The model under review builds one solid part; all positions refer to its coordinate system, in mm. A direction names the side the tool comes from. Coordinates: 2 decimals unless noted, no trailing zeros. Loops run counter-clockwise (first coordinate to the right, second up) from the corner with the lowest first, then second, coordinate; pieces in that order, holes last. Notation, with made-up numbers: M 16,84.5 L 68,84.5 A25 ccw 68,110.5 Z; hole C 68,0 d10. An arc over 180 degrees is marked long. Write item = value, one per line. Start each with the question number.
Q1. We need section A-A on y = 12. Give the boundary of the cut face in (x, z), and give its area (3 significant figures).
Q2. Clearance check with flat-ended pins moving along their axes: pin 1 Ø5.5 at (y, z) = (26, 26.5) entering from +X; pin 2 Ø4 at (y, z) = (21, -32) entering from -X; pin 3 Ø10.5 at (x, z) = (-17.5, 10) entering from +Y; pin 4 Ø2 at (x, y) = (-64, -3) entering from -Z. State where each tip first meets the part, or that it passes through.
Q3. Mouldability with a two-part tool opening along Z and no side actions: class faces 1 (the face through (24.5, 29.9, 9.8)), 2 (the face through (-65, -2, -27.5)), 3 (the face through (-26.577, 31.774, 32.535)) as released by +Z, released by -Z, zero draft, split by the parting line, or undercut.
Q4. Wall thickness on probe 1 along Y at (x, z) = (27.5, 32.55); probe 2 along X at (y, z) = (30, 33.95); probe 3 along X at (y, z) = (25, 22.5): over which ranges is each line inside the solid? List them lowest first.
Q5. We need section C-C on x = 9. Give the boundary of the cut face in (y, z), and give its area (3 significant figures).
Q6. We need section B-B on x = -69.5. Give the boundary of the cut face in (y, z), and give its area (3 significant figures).
Q7. We need section D-D on z = -7.5. Give the boundary of the cut face in (x, y), and give its area (3 significant figures).
Q8. For faces 4 (the face through (-27, 18, -30)), 5 (the face through (-24.5, 5.1, 9.8)), 6 (the face through (21.466, -2.535, 10.521)), 7 (the face through (-9, 5, 0)), list the 3-axis set-ups (+Z, -Z, +X, -X, +Y, -Y) from which the entire face can be reached by the end or side of a thin tool; tool diameter is ignored.
from build123d import *

# Parameters (mm, degrees)
SKETCH_1_W          = 45
SKETCH_1_H          = 70
SKETCH_1_R          = 21.5
EXTRUDE_1_DEPTH     = 35
SKETCH_2_R          = 21.5
EXTRUDE_2_DEPTH     = 5
SKETCH_3_R          = 2
SKETCH_3_R_2        = 13
CUT_EXTRUDE_1_DEPTH = 10
SKETCH_5_W          = 10
SKETCH_5_H          = 35
EXTRUDE_3_DEPTH     = 5
SKETCH_6_R          = 2
CUT_EXTRUDE_2_DEPTH = 5
EXTRUDE_START       = 5
SKETCH_8_R          = 22.5
SKETCH_8_R_2        = 13
SKETCH_8_R_3        = 2
EXTRUDE_5_DEPTH     = 5
SKETCH_9_R          = 4
CUT_EXTRUDE_3_DEPTH = 5
EXTRUDE_6_DEPTH     = 7
SKETCH_11_W         = 25
SKETCH_11_H         = 15
EXTRUDE_7_DEPTH     = 7
FILLET_1_R          = 4
SKETCH_12_R         = 2.5
CUT_EXTRUDE_4_DEPTH = 10
SKETCH_13_W         = 5
SKETCH_13_H         = 30
EXTRUDE_8_DEPTH     = 35
SKETCH_14_W         = 65
SKETCH_14_H         = 35
EXTRUDE_9_DEPTH     = 5
CUT_EXTRUDE_START   = -5
SKETCH_16_R         = 2
CUT_EXTRUDE_5_DEPTH = 5
SKETCH_18_R         = 3
CUT_EXTRUDE_6_DEPTH = 31


with BuildPart() as part:
    # 草图1 → 凸台-拉伸1 (new body)
    with BuildSketch(Plane(origin=(0, 0, 0), x_dir=(1, 0, 0), z_dir=(0, 1, 0))):
        Rectangle(SKETCH_1_W, SKETCH_1_H)
        with Locations(Location((0, -10, 0), (0, 0, 270))):
            Circle(SKETCH_1_R, mode=Mode.SUBTRACT)
    extrude(amount=EXTRUDE_1_DEPTH)

    # 草图2 → 凸台-拉伸2 (add)
    with BuildSketch(Plane.XZ):
        with Locations(Location((0, 10, 0), (0, 0, 270))):
            Circle(SKETCH_2_R)
    extrude(amount=-EXTRUDE_2_DEPTH)

    # 草图3 → 切除-拉伸1 (cut)
    with BuildSketch(Plane.XZ):
        with Locations(Location((0, -7.5, 0), (0, 0, 270))):
            Circle(SKETCH_3_R)
        with Locations(Location((-17.5, 10, 0), (0, 0, 270))):
            Circle(SKETCH_3_R)
        with Locations(Location((0, 27.5, 0), (0, 0, 270))):
            Circle(SKETCH_3_R)
        with Locations(Location((17.5, 10, 0), (0, 0, 270))):
            Circle(SKETCH_3_R)
        with Locations(Location((0, 10, 0), (0, 0, 270))):
            Circle(SKETCH_3_R_2)
    extrude(amount=-CUT_EXTRUDE_1_DEPTH, mode=Mode.SUBTRACT)

    # 草图5 → 凸台-拉伸3 (add)
    with BuildSketch(Plane(origin=(0, 0, -35), x_dir=(-1, 0, 0), z_dir=(0, 0, -1))):
        with Locations((27.5, 17.5)):
            Rectangle(SKETCH_5_W, SKETCH_5_H)
        with Locations((-27.5, 17.5)):
            Rectangle(SKETCH_5_W, SKETCH_5_H)
    extrude(amount=-EXTRUDE_3_DEPTH)

    # 草图6 → 切除-拉伸2 (cut)
    with BuildSketch(Plane.XY.offset(-30)):
        with Locations((27.5, 30)):
            Circle(SKETCH_6_R)
        with Locations((27.5, 5)):
            Circle(SKETCH_6_R)
        with Locations((-27.5, 30)):
            Circle(SKETCH_6_R)
        with Locations((-27.5, 5)):
            Circle(SKETCH_6_R)
    extrude(amount=-CUT_EXTRUDE_2_DEPTH, mode=Mode.SUBTRACT)

    # 草图8 → 凸台-拉伸5 (add)
    with BuildSketch(Plane.XZ.offset(EXTRUDE_START)):
        with Locations(Location((0, 10, 0), (0, 0, 180))):
            Circle(SKETCH_8_R)
        with Locations(Location((0, 10, 0), (0, 0, 270))):
            Circle(SKETCH_8_R_2, mode=Mode.SUBTRACT)
        with Locations(Location((-17.5, 10, 0), (0, 0, 270))):
            Circle(SKETCH_8_R_3, mode=Mode.SUBTRACT)
        with Locations(Location((0, -7.5, 0), (0, 0, 270))):
            Circle(SKETCH_8_R_3, mode=Mode.SUBTRACT)
        with Locations(Location((17.5, 10, 0), (0, 0, 270))):
            Circle(SKETCH_8_R_3, mode=Mode.SUBTRACT)
        with Locations(Location((0, 27.5, 0), (0, 0, 270))):
            Circle(SKETCH_8_R_3, mode=Mode.SUBTRACT)
    extrude(amount=-EXTRUDE_5_DEPTH)

    # 草图9 → 切除-拉伸3 (cut)
    with BuildSketch(Plane.XZ.offset(5)):
        with Locations(Location((0, 27.5, 0), (0, 0, 270))):
            Circle(SKETCH_9_R)
        with Locations(Location((-17.5, 10, 0), (0, 0, 270))):
            Circle(SKETCH_9_R)
        with Locations(Location((17.5, 10, 0), (0, 0, 270))):
            Circle(SKETCH_9_R)
        with Locations(Location((0, -7.5, 0), (0, 0, 270))):
            Circle(SKETCH_9_R)
    extrude(amount=-CUT_EXTRUDE_3_DEPTH, mode=Mode.SUBTRACT)

    # 草图10 → 凸台-拉伸6 (add)
    with BuildSketch(Plane.XZ.offset(5)):
        with BuildLine():
            Line((-19.899748742, 20.5), (-77, 20.5))
            Line((-77, 20.5), (-77, -12.5))
            Line((-77, -12.5), (0, -12.5))
            ThreePointArc((0, -12.5), (-19.267848868, -1.618950039), (-19.899748742, 20.5))
        make_face()
    extrude(amount=-EXTRUDE_6_DEPTH)

    # 草图11 → 凸台-拉伸7 (add)
    with BuildSketch(Plane.XZ.offset(5)):
        with Locations((-64.5, -20)):
            Rectangle(SKETCH_11_W, SKETCH_11_H)
    extrude(amount=-EXTRUDE_7_DEPTH)

    # 圆角1
    fillet_1_edges = [part.edges().sort_by_distance(p)[0] for p in [
        (-77, -1.5, 20.5),
        (-77, -1.5, -27.5),
        (-52, -1.5, -12.5),
        (-52, -1.5, -27.5),
    ]]
    fillet(fillet_1_edges, radius=FILLET_1_R)

    # 草图12 → 切除-拉伸4 (cut)
    with BuildSketch(Plane.XZ.offset(5)):
        with Locations(Location((-69.5, -15, 0), (0, 0, 270))):
            Circle(SKETCH_12_R)
        with Locations(Location((-69.5, 15, 0), (0, 0, 270))):
            Circle(SKETCH_12_R)
    extrude(amount=-CUT_EXTRUDE_4_DEPTH, mode=Mode.SUBTRACT)

    # 草图13 → 凸台-拉伸8 (add)
    with BuildSketch(Plane(origin=(0, 0, 0), x_dir=(1, 0, 0), z_dir=(0, 1, 0))):
        with Locations((25, -10)):
            Rectangle(SKETCH_13_W, SKETCH_13_H)
        with Locations((-25, -10)):
            Rectangle(SKETCH_13_W, SKETCH_13_H)
    extrude(amount=EXTRUDE_8_DEPTH)

    # 草图14 → 凸台-拉伸9 (add)
    with BuildSketch(Plane.XY.offset(35)):
        with Locations((0, 17.5)):
            Rectangle(SKETCH_14_W, SKETCH_14_H)
    extrude(amount=-EXTRUDE_9_DEPTH)

    # 草图16 → 切除-拉伸5 (cut)
    with BuildSketch(Plane(origin=(0, 0, 30), x_dir=(-1, 0, 0), z_dir=(0, 0, -1)).offset(CUT_EXTRUDE_START)):
        with Locations(Location((-27.5, 30, 0), (0, 0, 180))):
            Circle(SKETCH_16_R)
        with Locations(Location((-27.5, 5, 0), (0, 0, 180))):
            Circle(SKETCH_16_R)
        with Locations(Location((27.5, 30, 0), (0, 0, 180))):
            Circle(SKETCH_16_R)
        with Locations(Location((27.5, 5, 0), (0, 0, 180))):
            Circle(SKETCH_16_R)
    extrude(amount=CUT_EXTRUDE_5_DEPTH, mode=Mode.SUBTRACT)

    # 草图18 → 切除-拉伸6 (cut)
    with BuildSketch(Plane(origin=(0, 0, -5), x_dir=(-1, 0, 0), z_dir=(0, 0, -1))):
        with Locations((27.5, 30)):
            Circle(SKETCH_18_R)
        with Locations((27.5, 5)):
            Circle(SKETCH_18_R)
        with Locations((-27.5, 5)):
            Circle(SKETCH_18_R)
        with Locations((-27.5, 30)):
            Circle(SKETCH_18_R)
    extrude(amount=-CUT_EXTRUDE_6_DEPTH, mode=Mode.SUBTRACT)


solid = part.part
Returned:
q1.outline = M -32.5,-35 L 32.5,-35 L 32.5,-30 L 22.5,-30 L 22.5,-5 L 27.5,-5 L 27.5,25 L 22.5,25 L 22.5,30 L 32.5,30 L 32.5,35 L -32.5,35 L -32.5,30 L -22.5,30 L -22.5,25 L -27.5,25 L -27.5,-5 L -22.5,-5 L -22.5,-30 L -32.5,-30 Z; hole M -7.89,30 A21.5 ccw long 7.89,30 Z
q1.area = 2,210 mm^2
q2.pin_1 = 27.5
q2.pin_2 = -32.5
q2.pin_3 = 35
q2.pin_4 = -27.5
q3.face_1 = undercut
q3.face_2 = released by -Z
q3.face_3 = zero draft
q4.probe_1 = 0 to 3, 7 to 28, 32 to 35
q4.probe_2 = -32.5 to -29.5, -25.5 to 25.5, 29.5 to 32.5
q4.probe_3 = -27.5 to -17.49, 17.49 to 27.5
q5.outline = M -5,-10.62 L 0,-10.62 L 0,-35 L 35,-35 L 35,-9.53 L 5,-9.53 L 5,0.62 L -5,0.62 Z; M -5,19.38 L 5,19.38 L 5,29.53 L 35,29.53 L 35,35 L 0,35 L 0,30.62 L -5,30.62 Z
q5.area = 1,300 mm^2
q6.outline = M -5,-27.5 L 2,-27.5 L 2,-17.5 L -5,-17.5 Z; M -5,-12.5 L 2,-12.5 L 2,12.5 L -5,12.5 Z; M -5,17.5 L 2,17.5 L 2,20.5 L -5,20.5 Z
q6.area = 266 mm^2
q7.outline = M -77,-5 L -4,-5 L -4,0 L -2,0 L -2,5 L -12.49,5 L -12.49,35 L -22.5,35 L -22.5,2 L -77,2 Z; M 2,0 L 4,0 L 4,-5 L 14.14,-5 L 14.14,0 L 22.5,0 L 22.5,35 L 12.49,35 L 12.49,5 L 2,5 Z
q7.area = 1,330 mm^2
q8.face_4 = -X, +Y, -Y
q8.face_5 = -X
q8.face_6 = -Y
q8.face_7 = +Y
